```python
from build123d import *

# Parameters (mm, degrees)
F1_DEPTH    = 13.25
F2_DEPTH    = 13.25
F3_R        = 1
F4_R        = 1.99999
F5_T1_DEPTH = 26.5
F6_R        = 4
F7_SIZE     = 2
F8_R        = 4
F9_R        = 2
F10_R       = 0.5


# Not quite as in the source:
# - a fillet or chamfer that OpenCascade refuses, or shapes differently, is made with other operations: its cross-section is extruded or revolved along the edge and cut away or added
# - a fillet or chamfer is up to 0.001 mm smaller than in the source, because OpenCascade refuses the exact size


with BuildPart() as f1:
    # F0 (on Right) → F1 (new body, symmetric)
    with BuildSketch(Plane.YZ):
        with BuildLine():
            Line((24.5604159161, 8.2188727885), (-25.0402941419, 31.3480637385))
            Line((-25.0402941419, 31.3480637385), (-27.5760037124, 25.9102170163))
            Line((-27.5760037124, 25.9102170163), (-23.9507725642, 24.2197439694))
            Line((-23.9507725642, 24.2197439694), (-23.1055360408, 26.0323595434))
            Line((-23.1055360408, 26.0323595434), (-12.7312477201, 21.1947494516))
            Line((-12.7312477201, 21.1947494516), (-10.9610116945, 20.3692748361))
            Line((-10.9610116945, 20.3692748361), (4.9900053574, 12.9311934295))
            Line((4.9900053574, 12.9311934295), (6.760241383, 12.105718814))
            Line((6.760241383, 12.105718814), (7.7089287185, 11.6633386442))
            Line((7.7089287185, 11.6633386442), (15.0956095835, 8.2188727885))
            Line((15.0956095835, 8.2188727885), (7.7089287185, 8.2188727885))
            Line((7.7089287185, 8.2188727885), (-20.8974118188, 8.2188727885))
            ThreePointArc((-20.8974118188, 8.2188727885), (-26.4974118188, 2.6188727885), (-20.8974118188, -2.9811272115))
            Line((-20.8974118188, -2.9811272115), (30.894998731, -2.9811272115))
            ThreePointArc((30.894998731, -2.9811272115), (30.580160342, -1.8806088655), (29.580710732, -1.3226085804))
            Line((29.580710732, -1.3226085804), (16.8007476451, 0.2188727885))
            Line((16.8007476451, 0.2188727885), (6.4900759503, 0.2188727885))
            Line((6.4900759503, 0.2188727885), (-14.5099240497, 0.2188727885))
            ThreePointArc((-14.5099240497, 0.2188727885), (-16.5099240497, 2.2188727885), (-14.5099240497, 4.2188727885))
            Line((-14.5099240497, 4.2188727885), (24.5604159161, 4.2188727885))
            ThreePointArc((24.5604159161, 4.2188727885), (25.8345564377, 6.2188727885), (24.5604159161, 8.2188727885))
        make_face()
        Polygon((-10.9610116945, 20.3692748361), (-12.7312477201, 21.1947494516), (-11.7561154197, 15.664499365), (1.8970210747, 9.2979372598), (6.760241383, 12.105718814), (4.9900053574, 12.9311934295), (1.8183399389, 11.1000315463), (-10.3250558464, 16.762589997), align=None)
    extrude(amount=F1_DEPTH, both=True)

    # F0 (on Right) → F2 (join, symmetric)
    with BuildSketch(Plane.YZ):
        with BuildLine():
            Line((15.0956095835, 8.2188727885), (7.7089287185, 11.6633386442))
            ThreePointArc((7.7089287185, 11.6633386442), (8.806112099, 9.9411057164), (7.7089287185, 8.2188727885))
            Line((7.7089287185, 8.2188727885), (15.0956095835, 8.2188727885))
        make_face()
        with BuildLine():
            Line((24.5604159161, 8.2188727885), (-25.0402941419, 31.3480637385))
            Line((-25.0402941419, 31.3480637385), (-27.5760037124, 25.9102170163))
            Line((-27.5760037124, 25.9102170163), (-23.9507725642, 24.2197439694))
            Line((-23.9507725642, 24.2197439694), (-23.1055360408, 26.0323595434))
            Line((-23.1055360408, 26.0323595434), (-12.7312477201, 21.1947494516))
            Line((-12.7312477201, 21.1947494516), (-10.9610116945, 20.3692748361))
            Line((-10.9610116945, 20.3692748361), (4.9900053574, 12.9311934295))
            Line((4.9900053574, 12.9311934295), (6.760241383, 12.105718814))
            Line((6.760241383, 12.105718814), (7.7089287185, 11.6633386442))
            Line((7.7089287185, 11.6633386442), (15.0956095835, 8.2188727885))
            Line((15.0956095835, 8.2188727885), (7.7089287185, 8.2188727885))
            Line((7.7089287185, 8.2188727885), (-20.8974118188, 8.2188727885))
            ThreePointArc((-20.8974118188, 8.2188727885), (-26.4974118188, 2.6188727885), (-20.8974118188, -2.9811272115))
            Line((-20.8974118188, -2.9811272115), (30.894998731, -2.9811272115))
            ThreePointArc((30.894998731, -2.9811272115), (30.580160342, -1.8806088655), (29.580710732, -1.3226085804))
            Line((29.580710732, -1.3226085804), (16.8007476451, 0.2188727885))
            Line((16.8007476451, 0.2188727885), (6.4900759503, 0.2188727885))
            Line((6.4900759503, 0.2188727885), (-14.5099240497, 0.2188727885))
            ThreePointArc((-14.5099240497, 0.2188727885), (-16.5099240497, 2.2188727885), (-14.5099240497, 4.2188727885))
            Line((-14.5099240497, 4.2188727885), (24.5604159161, 4.2188727885))
            ThreePointArc((24.5604159161, 4.2188727885), (25.8345564377, 6.2188727885), (24.5604159161, 8.2188727885))
        make_face()
        Polygon((7.5313132472, 1.2188727885), (6.4900759503, 0.2188727885), (16.8007476451, 0.2188727885), align=None)
    extrude(amount=F2_DEPTH, both=True)

    # F3
    f3_edges = [f1.edges().sort_by_distance(p)[0] for p in [
        (0, 6.490076, 0.218873),
        (0, 7.531313, 1.218873),
        (0, 16.800748, 0.218873),
    ]]
    fillet(f3_edges, radius=F3_R)

    # F4 (radius 2 in the source; OpenCascade refuses exactly that, so slightly less here)
    f4_edges = [f1.edges().sort_by_distance(p)[0] for p in [
        (0, -23.105536, 26.03236),
        (0, 24.560416, 8.218873),
        (0, 24.560416, 4.218873),
        (0, 7.708929, 8.218873),
        (0, 7.708929, 11.663339),
    ]]
    fillet(f4_edges, radius=F4_R)

    # F5: fillet of radius 5 on 2 edges, made by hand

    # F5_s2 → F5_t1 (join)
    with BuildSketch(Plane.YZ.offset(-13.25)):
        with BuildLine():
            ThreePointArc((-12.2792701217, 18.6314571149), (-13.2365421853, 20.8070233716), (-15.090217578, 22.2947551617))
            Line((-15.090217578, 22.2947551617), (-12.7312477201, 21.1947494516))
            Line((-12.7312477201, 21.1947494516), (-12.2792701217, 18.6314571149))
        make_face()
        with BuildLine():
            ThreePointArc((6.9194699805, 12.0314692995), (6.3536054599, 11.8292518467), (5.8160865891, 11.5606107896))
            Line((5.8160865891, 11.5606107896), (6.760241383, 12.105718814))
            Line((6.760241383, 12.105718814), (6.9194699805, 12.0314692995))
        make_face()
    extrude(amount=F5_T1_DEPTH)

    # F6
    f6_edges = [f1.edges().sort_by_distance(p)[0] for p in [
        (0, 1.897021, 9.297937),
        (0, -11.756115, 15.664499),
    ]]
    fillet(f6_edges, radius=F6_R)

    # F7
    f7_edges = [f1.edges().sort_by_distance(p)[0] for p in [
        (13.25, -2.985503, 16.650234),
        (-13.25, -2.985503, 16.650234),
    ]]
    chamfer(f7_edges, length=F7_SIZE)

    # F8
    f8_edges = [f1.edges().sort_by_distance(p)[0] for p in [
        (-11.25, -2.985503, 16.650234),
        (11.25, -2.985503, 16.650234),
    ]]
    fillet(f8_edges, radius=F8_R)

    # F9
    f9_edges = [f1.edges().sort_by_distance(p)[0] for p in [
        (0, -10.325056, 16.76259),
        (0, 1.81834, 11.100032),
    ]]
    fillet(f9_edges, radius=F9_R)

    # F10
    f10_edges = [f1.edges().sort_by_distance(p)[0] for p in [
        (-11.167025, 5.331118, 13.128135),
        (-11.167025, -11.029409, 20.757174),
        (11.123879, -11.025557, 20.735332),
        (0, -10.961012, 20.369275),
        (11.123879, 5.31191, 13.117045),
        (0, 4.990005, 12.931193),
    ]]
    fillet(f10_edges, radius=F10_R)


solid = f1.part
```
Work out the finished part from the listing and answer in its coordinate system (mm). A direction names the side the tool comes from. Round coordinates to 2 decimals unless told otherwise and drop trailing zeros. Loops run counter-clockwise (first coordinate to the right, second up) from the corner with the lowest first, then second, coordinate; pieces in that order, holes last. Notation, with made-up numbers: M 20.5,76.25 L 71.5,76.25 A18 cw 71.5,107.25 Z; hole C 88.25,66 d9. An arc over 180 degrees is marked long. One line per question, with ' | ' between items.
Q1. Consider line 1 along Z through (x, y) = (-1, -5); line 2 along Z through (x, y) = (-7, -13); line 3 along Z through (x, y) = (8, 7.5). Determine where each line is inside the solid, lowest interval first. Write a range as from..to.
Conclusion:
line 1: z = -2.98..0.22, 4.22..8.22, 12.51..14.28, 17.59..22 | line 2: z = -2.98..0.22, 4.22..8.22, 20.47..25.73 | line 3: z = -2.98..1.1, 4.22..8.82, 11.62..16.17
Q2. A tool of negligible diameter and unlimited length cuts with its end or side. For faces 1 (the flat face through (0.185, -4.182, 13.898)), 2 (the cylindrical face through (11.104, -2.749, 16.867)), 3 (the flat face through (0.185, -4.999, 12.513)), 4 (the cylindrical face through (0.19, 25.5, 7.39)), 5 (the flat face through (0.185, 23.28, -0.563)), from which of +Z, -Z, +X, -X, +Y, -Y can it reach the whole face along a straight path? Write none if from no direction.
Conclusion:
face 1: +X, -X | face 2: +X | face 3: +X, -X, -Y | face 4: +Z, +X, -X, +Y | face 5: +X, -X, +Y
Q3. Each of these flat-tipped pins is pushed along its axis until it touches: pin 1 Ø4 at (x, z) = (-4.5, 24) entering from +Y; pin 2 Ø3 at (x, y) = (-6.5, -19.5) entering from +Z; pin 3 Ø2 at (x, z) = (-3.5, 11.5) entering from +Y. Where does it stop, or does it pass through?
Conclusion:
pin 1: stops at y = -4.99 | pin 2: stops at z = 29.46 | pin 3: stops at y = 19.67
Q4. Find section B-B, the plane y = 12.5. Give the vertices of the cut face in (x, z).
Conclusion:
outline: M -13.25,-2.98 L 13.25,-2.98 L 13.25,0.68 L -13.25,0.68 Z; M -13.25,4.22 L 13.25,4.22 L 13.25,13.84 L -13.25,13.84 Z
Q5. Find section D-D, the plane z = 3.5. Give the vertices of the cut face in (x, y), then the cut area to 3 significant figures.
Conclusion:
outline: M -13.25,-26.43 L 13.25,-26.43 L 13.25,-16.05 L -13.25,-16.05 Z | area: 275 mm2
Q6. The mould has two halves that part along Z. Classify faces 6 (the cylindrical face through (-11.14, -2.74, 16.88)), 7 (the flat face through (0, 5, -2.981)), 8 (the flat face through (-13.25, -3, 7)): +Z half, -Z half, draft (parallel to the pull), parting line (faces both ways), or undercut.
Conclusion:
face 6: undercut | face 7: -Z half | face 8: draft
Q7. Find section A-A, the plane y = -23. Give the vertices of the cut face in (x, z), then the cut area to 3 significant figures.
Conclusion:
outline: M -13.25,-2.57 L 13.25,-2.57 L 13.25,7.81 L -13.25,7.81 Z; M -13.25,25.18 L 13.25,25.18 L 13.25,30.4 L -13.25,30.4 Z | area: 413 mm2
Q8. Find section C-C, the plane y = 26.5. Give the vertices of the cut face in (x, z), then the cut area to 3 significant figures.
Conclusion:
outline: M -13.25,-2.98 L 13.25,-2.98 L 13.25,-0.95 L -13.25,-0.95 Z | area: 53.8 mm2
